Source: CAD feature listing. Evaluate the final solid. Frame: model axes, mm. A direction names the side the tool comes from. Give positions to 0.01 mm unless a question says otherwise; leave off trailing zeros. Order: outer loops, then holes, each group sorted by start corner. A loop starts at its lowest first (then second) coordinate and runs counter-clockwise, first axis right, second up. Notation, with made-up numbers: M -24.75,41.5 L -0.75,41.5 A12 ccw -0.75,59.5 Z; hole C -39.75,13.5 d6. An arc over 180 degrees is marked long. One line per question, with ' | ' between items. Start each with the question number.
from build123d import *

# Parameters (mm, degrees)
F0_W     = 127
F0_H     = 266.7
F0_W_2   = 4.5
F0_H_2   = 12.7
F1_DEPTH = 4.826


with BuildPart() as f1:
    # F0 (on Front) → F1 (new body)
    with BuildSketch(Plane.XZ):
        with Locations((0, 32.769812)):
            Rectangle(F0_W, F0_H)
        with Locations((-59.054758, -56.475502)):
            Rectangle(F0_W_2, F0_H_2, mode=Mode.SUBTRACT)
        Polygon((-43.104758, -62.849627), (-43.104758, -50.149627), (-38.554112, -50.085164), (-38.554112, -62.849627), align=None, mode=Mode.SUBTRACT)
        Polygon((38.655718, -50.03741), (43.001247, -50.149624), (43.155718, -62.73741), (38.655718, -62.73741), align=None, mode=Mode.SUBTRACT)
        Polygon((56.856852, -62.745742), (56.701028, -50.047654), (61.304758, -50.125502), (61.304758, -62.825502), align=None, mode=Mode.SUBTRACT)
        with Locations((-59.054758, 122.015126)):
            Rectangle(F0_W_2, F0_H_2, mode=Mode.SUBTRACT)
        with Locations((-29.454758, 122.229226)):
            Rectangle(F0_W_2, F0_H_2, mode=Mode.SUBTRACT)
        with Locations((29.454758, 122.229226)):
            Rectangle(F0_W_2, F0_H_2, mode=Mode.SUBTRACT)
        with Locations((59.054758, 122.015126)):
            Rectangle(F0_W_2, F0_H_2, mode=Mode.SUBTRACT)
    extrude(amount=F1_DEPTH)


solid = f1.part
Item 1: Reachability of faces 1 (the flat face through (-59, -2, -62.826)), 2 (the flat face through (-1, -4.826, 35)) from +Z, -Z, +X, -X, +Y, -Y: full face, straight path, thin tool, end or side. Return the list, or none.
Item 2: Line query: line 1 (X direction, y = -0.6, z = -53); line 2 (Z direction, x = -57, y = -2.6); line 3 (X direction, y = -1.25, z = -60). Output: solid intervals per line, ascending.
Item 3: Cut plane A-A on z = 124. Return the cut outline in (x, y), and give its area (3 significant figures).
Item 4: Mould query, pull axis Z, two halves, no side actions, for faces 3 (the flat face through (-1, -2, -100.58)), 4 (the flat face through (59, -2, 115.665)), 5 (the flat face through (-63.5, -2, 31)). Classes: pulls with the +Z half, pulls with the -Z half, needs draft (parallel to the pull), parting line crosses it, or undercut.
Results are:
1) face 1: +Y, -Y | face 2: +Z, -Z, +X, -X, -Y
2) line 1: x = -63.5 to -61.3, -56.8 to -43.1, -38.55 to 38.66, 43.04 to 56.74, 61.3 to 63.5 | line 2: z = -100.58 to -62.83, -50.13 to 115.67, 128.37 to 166.12 | line 3: x = -63.5 to -61.3, -56.8 to -43.1, -38.55 to 38.66, 43.12 to 56.82, 61.3 to 63.5
3) outline: M -63.5,-4.83 L -61.3,-4.83 L -61.3,0 L -63.5,0 Z; M -56.8,-4.83 L -31.7,-4.83 L -31.7,0 L -56.8,0 Z; M -27.2,-4.83 L 27.2,-4.83 L 27.2,0 L -27.2,0 Z; M 31.7,-4.83 L 56.8,-4.83 L 56.8,0 L 31.7,0 Z; M 61.3,-4.83 L 63.5,-4.83 L 63.5,0 L 61.3,0 Z | area: 526 mm2
4) face 3: pulls with the -Z half | face 4: undercut | face 5: needs draft
